Read the model definition and answer for the solid it produces. Units are mm, in the model's axes. A direction names the side the tool comes from. Coordinates: 2 decimals unless noted, no trailing zeros. Write each loop counter-clockwise with the first axis right and the second up, starting at its lowest first coordinate (ties: lowest second). Pieces come first, ordered by that corner, then holes.
(1) Given pin 1 (1.5 mm diameter, centred on x = 23, z = 9.5, fed in from -Y); pin 2 (2 mm diameter, centred on x = 69.5, z = 6, fed in from -Y); pin 3 (4 mm diameter, centred on x = 112, z = 11.5, fed in from -Y), each flat-ended and moving along its own axis, determine where each tip first touches the part or whether it passes through.
(2) The part is cut by section C-C, the plane y = -20. Determine the outline of the cut face in (x, z).
(3) Which of the six approach directions +Z, -Z, +X, -X, +Y, -Y give full straight-line access (tool end or side, diameter ignored) to faces 1 (the flat face through (95, -38.951, 13)), 2 (the flat face through (76.2, 0, 13)), 3 (the flat face through (27, -62, 25.4))?
(4) The part is cut by section A-A, the plane y = -50. Determine the outline of the cut face in (x, z).
(5) The part is cut by section D-D, the plane x = 7. Determine the outline of the cut face in (y, z), and give its area (3 significant figures).
(6) The part is cut by section B-B, the plane z = 6.5. Determine the outline of the cut face in (x, y), and give its area (3 significant figures).
(7) Determine the mould class of faces 4 (the cylindrical face through (126.441, -64.345, 12.522)), 5 (the flat face through (-50.8, 0, 13)), 6 (the flat face through (152.4, -1, 13)), 7 (the flat face through (6, -38.951, 13)) for opening direction X: pulls with the +X half, pulls with the -X half, needs draft (parallel to the pull), parting line crosses it, or undercut.
(8) Straight lines are drawn through the part: line 1 along X through (y, z) = (8, 3); line 2 along X through (y, z) = (-57, 2); line 3 along X through (y, z) = (-44.5, 16.5). For each, find the intervals that lie inside material, in ascending order.
```python
from build123d import *

# Parameters (mm, degrees)
F1_DEPTH = 25.4


with BuildPart() as f1:
    # F0 (on Top) → F1 (new body)
    with BuildSketch(Plane.XY):
        with BuildLine():
            Line((25.4, 37.248519), (-50.8, 37.248519))
            Line((-50.8, 37.248519), (-50.8, -38.951481))
            ThreePointArc((-50.8, -38.951481), (-25.4, -64.351481), (0, -38.951481))
            Line((0, -38.951481), (12.7, -38.951481))
            Line((12.7, -38.951481), (12.7, -89.751481))
            ThreePointArc((12.7, -89.751481), (23.859232, -116.692249), (50.8, -127.851481))
            ThreePointArc((50.8, -127.851481), (77.740768, -116.692249), (88.9, -89.751481))
            Line((88.9, -89.751481), (88.9, -38.951481))
            Line((88.9, -38.951481), (101.6, -38.951481))
            ThreePointArc((101.6, -38.951481), (127, -64.351481), (152.4, -38.951481))
            Line((152.4, -38.951481), (152.4, 37.248519))
            Line((152.4, 37.248519), (76.2, 37.248519))
            Line((76.2, 37.248519), (76.2, -38.951481))
            ThreePointArc((76.2, -38.951481), (68.760512, -56.911993), (50.8, -64.351481))
            ThreePointArc((50.8, -64.351481), (32.839488, -56.911993), (25.4, -38.951481))
            Line((25.4, -38.951481), (25.4, 37.248519))
        make_face()
    extrude(amount=F1_DEPTH)


solid = f1.part
```
Computed:
1. pin 1: stops at y = -116.58
1. pin 2: stops at y = -123.49
1. pin 3: stops at y = -60.77
2. outline: (-50.8, 0) - (25.4, 0) - (25.4, 25.4) - (-50.8, 25.4) - close; (76.2, 0) - (152.4, 0) - (152.4, 25.4) - (76.2, 25.4) - close
3. face 1: +Z, -Z, -Y
3. face 2: +Z, -Z, +Y
3. face 3: +Z, +X, -X, +Y, -Y
4. outline: (-48.27, 0) - (-2.53, 0) - (-2.53, 25.4) - (-48.27, 25.4) - close; (12.7, 0) - (27.93, 0) - (27.93, 25.4) - (12.7, 25.4) - close; (73.67, 0) - (88.9, 0) - (88.9, 25.4) - (73.67, 25.4) - close; (104.13, 0) - (149.87, 0) - (149.87, 25.4) - (104.13, 25.4) - close
5. outline: (-38.95, 0) - (37.25, 0) - (37.25, 25.4) - (-38.95, 25.4) - close
5. area: 1,940 mm2
6. outline: (-50.8, -38.95) arc R25.4 ccw to (0, -38.95) - (12.7, -38.95) - (12.7, -89.75) arc R38.1 ccw to (50.8, -127.85) arc R38.1 ccw to (88.9, -89.75) - (88.9, -38.95) - (101.6, -38.95) arc R25.4 ccw to (152.4, -38.95) - (152.4, 37.25) - (76.2, 37.25) - (76.2, -38.95) arc R25.4 cw to (50.8, -64.35) arc R25.4 cw to (25.4, -38.95) - (25.4, 37.25) - (-50.8, 37.25) - close
6. area: 18,800 mm2
7. face 4: undercut
7. face 5: pulls with the -X half
7. face 6: pulls with the +X half
7. face 7: undercut
8. line 1: x = -50.8 to 25.4, 76.2 to 152.4
8. line 2: x = -43.27 to -7.53, 12.7 to 32.93, 68.67 to 88.9, 109.13 to 144.87
8. line 3: x = -50.19 to -0.61, 12.7 to 26.01, 75.59 to 88.9, 102.21 to 151.79
